from build123d import *

# Parameters (mm, degrees)
F1_DEPTH = 1219.2
F3_DEPTH = 38.101


with BuildPart() as f1:
    # F0 (on Front) → F1 (new body)
    with BuildSketch(Plane.XZ):
        Polygon((0, 38.1), (0, 0), (38.1, 0), (38.1, 4.7625), (4.7625, 4.7625), (4.7625, 38.1), align=None)
    extrude(amount=F1_DEPTH)

    # F2 (on face) → F3 (cut, through all)
    with BuildSketch(Plane(origin=(0, 0, 0), x_dir=(0, -1, 0), z_dir=(-1, 0, 0))):
        Polygon((1181.1, 38.1), (1219.2, 0), (1219.2, 38.1), align=None)
        Polygon((0, 0), (38.1, 38.1), (0, 38.1), align=None)
    extrude(amount=-F3_DEPTH, mode=Mode.SUBTRACT)


solid = f1.part
Design review of the part built by this model. Coordinates are the model's own, in mm. A direction names the side the tool comes from. Give positions to 0.01 mm unless a question says otherwise; leave off trailing zeros. Loops run counter-clockwise (first coordinate to the right, second up) from the corner with the lowest first, then second, coordinate; pieces in that order, holes last. Notation, with made-up numbers: M 65.25,-19.5 L 89.25,-19.5 A27 cw 89.25,17.5 Z; hole C -10,1.25 d1. An arc over 180 degrees is marked long. One line per question, with ' | ' between items. Start each with the question number.
1. To check wall thickness, follow L1, parallel to Z at x = 31, y = -1009.5; L2, parallel to Y at x = 14.5, z = 2.5. State the ranges of each line that lie inside material, in increasing order.
2. Add section B-B (z = 25.5). Write out the cut boundary in (x, y).
3. Insertion check: P1, Ø10, axis at y = -808, z = 29.5, coming from the +X side; P2, Ø1, axis at x = 6.5, z = 27, coming from the -Y side (3 decimals); P3, Ø16.5, axis at x = 29.5, y = -504, coming from the +Z side. Each pin has a flat end and moves straight along its axis. Give the tip position at first contact, or say it passes through.
4. For faces 1 (the face through (19, -601, 0)), 2 (the face through (22, -601, 4.762)), list the 3-axis set-ups (+Z, -Z, +X, -X, +Y, -Y) from which the entire face can be reached by the end or side of a thin tool; tool diameter is ignored.
5. Add section C-C (x = 28.5). Write out the cut boundary in (y, z).
6. Add section A-A (y = -418). Write out the cut boundary in (x, z).
Worked out:
1) L1: z = 0 to 4.76 | L2: y = -1216.7 to -2.5
2) outline: M 0,-1193.7 L 4.76,-1193.7 L 4.76,-25.5 L 0,-25.5 Z
3) P1: stops at x = 4.76 | P2: passes through | P3: stops at z = 4.76
4) face 1: -Z, +X, -X, +Y, -Y | face 2: +Z, +X, +Y, -Y
5) outline: M -1219.2,0 L 0,0 L -4.76,4.76 L -1214.44,4.76 Z
6) outline: M 0,0 L 38.1,0 L 38.1,4.76 L 4.76,4.76 L 4.76,38.1 L 0,38.1 Z
